Check sheet for the modelled part. Datum: model origin and axes. Units: mm. Face numbers are marked on the shaded views. A direction names the side the tool comes from. Coordinates: 2 decimals unless noted, no trailing zeros. Loops run counter-clockwise (first coordinate to the right, second up) from the corner with the lowest first, then second, coordinate; pieces in that order, holes last. Notation, with made-up numbers: (75.5, -1) - (91.5, -1) arc R18 cw to (91.5, 27) - close; hole circle Ø10 at (2, 0.5). An arc over 180 degrees is marked (long way). Use a Markdown table: item, result. Add a question column.
1) Sectioned sample at D-D, the plane x = 5.5. Enter the section's corners in (y, z).
2) Thickness scan on line 1 (X direction, y = -10.5, z = -4); line 2 (Y direction, x = 29, z = -2); line 3 (X direction, y = -14, z = -20). Record the ranges inside material, lowest first.
3) Sectioned sample at B-B, the plane z = -7. Enter the section's corners in (x, y), then the cut area to 3 significant figures.
4) Draft check along Z on the marked faces 1, 2 and 3. Enter one of: pulls with the +Z half, pulls with the -Z half, needs draft (parallel to the pull), parting line crosses it, or undercut.
5) Sectioned sample at C-C, the plane y = -8. State how many separate pieces and enclosed holes the cut face has, then the cut area to 3 significant figures.
6) Sectioned sample at A-A, the plane y = -16.5. Enter the section's corners in (x, z), then the cut area to 3 significant figures.
7) Tool access check on the marked faces 4, 5, 6 and 7. Record the directions out of +Z, -Z, +X, -X, +Y, -Y that give a thin tool (end or side, any length) a straight path to the whole face; none if there is none.
8) Go/stop test with flat-tipped pins: P1, Ø1.5, axis at x = -23, y = -9.5, coming from the +Z side; P2, Ø9.5, axis at x = 16, z = 0.5, coming from the -Y side; P3, Ø16.5, axis at x = 7.5, y = -5.5, coming from the -Z side. Record where each tip stops, or that it passes through.
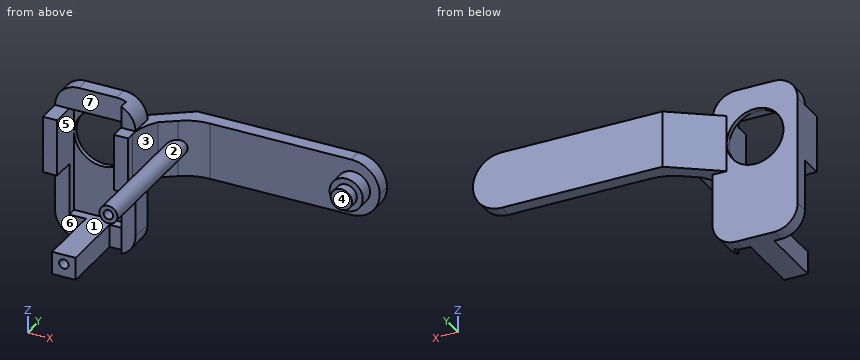
from build123d import *

# Parameters (mm, degrees)
SKETCH1_W            = 40
SKETCH1_H            = 12
BOSS_EXTRUDE1_DEPTH  = 3
SKETCH1_7_R          = 3.5
BOSS_EXTRUDE2_DEPTH  = 3
BOSS_EXTRUDE4_DEPTH  = 12
SKETCH4_W            = 3
SKETCH4_H            = 12
BOSS_EXTRUDE5_DEPTH  = 5
FILLET3_R            = 10
BOSS_EXTRUDE11_START = -27.8
BOSS_EXTRUDE11_DEPTH = 32.8
CUT_EXTRUDE2_DEPTH   = 47.899705007
FILLET7_R            = 6
BOSS_EXTRUDE12_DEPTH = 5
CUT_EXTRUDE3_START   = -2
CUT_EXTRUDE3_DEPTH   = 2
SKETCH13_W           = 3
SKETCH13_H           = 12
BOSS_EXTRUDE13_DEPTH = 5
SKETCH13_3_W         = 5
SKETCH13_3_H         = 4.8
BOSS_EXTRUDE14_DEPTH = 14
SKETCH14_R           = 1
CUT_EXTRUDE4_DEPTH   = 10
FILLET8_R            = 10
FILLET9_R            = 5
SKETCH15_R           = 1.9
SKETCH15_R_2         = 1
BOSS_EXTRUDE15_DEPTH = 30
SKETCH15_2_R         = 1
BOSS_EXTRUDE16_DEPTH = 20


# Read off the part's stored shape, not the designer's step: Boss-Extrude11, Cut-Extrude3
# Some blends are built 0.0001 mm under size
with BuildPart() as part:
    # Sketch1 → Boss-Extrude1 (new body)
    with BuildSketch(Plane(origin=(0, 0, 0), x_dir=(1, 0, 0), z_dir=(0, 1, 0))):
        with Locations((20.375241408, -0.133846421)):
            Rectangle(SKETCH1_W, SKETCH1_H)
    extrude(amount=BOSS_EXTRUDE1_DEPTH)

    # Sketch1<7> → Boss-Extrude2 (add)
    with BuildSketch(Plane(origin=(0, 0, 0), x_dir=(1, 0, 0), z_dir=(0, 1, 0))):
        with Locations(Location((34.817424324, -0.133846421, 0), (0, 0, 270))):
            Circle(SKETCH1_7_R)
    extrude(amount=-BOSS_EXTRUDE2_DEPTH)

    # Sketch3 → Boss-Extrude4 (add)
    with BuildSketch(Plane.XY.offset(6.133846421)):
        Polygon((0.375241408, 3), (-9.624758592, -4), (-4.393377613, -4), (5.606622387, 3), align=None)
    extrude(amount=-BOSS_EXTRUDE4_DEPTH)

    # Sketch4 → Boss-Extrude5 (add)
    with BuildSketch(Plane(origin=(0, -4, 0), x_dir=(-1, 0, 0), z_dir=(0, -1, 0))):
        with Locations((8.124758592, -0.133846421)):
            Rectangle(SKETCH4_W, SKETCH4_H)
    extrude(amount=BOSS_EXTRUDE5_DEPTH)

    # Fillet3
    fillet3_edges = [part.edges().sort_by_distance(p)[0] for p in [
        (1.320908101, 0, 0.133846421),
    ]]
    fillet(fillet3_edges, radius=FILLET3_R)

    # Boss-Extrude11 outline → Boss-Extrude11 (add)
    with BuildSketch(Plane.XY.offset(6.133846421).offset(BOSS_EXTRUDE11_START)):
        Polygon((-9.624758592, -7), (-9.624758592, -9), (-6.624758592, -9), (-6.624758592, -4), (-24.624758592, -4), (-24.624758592, -7), align=None)
    extrude(amount=BOSS_EXTRUDE11_DEPTH)

    # Sketch12 → Cut-Extrude2 (cut, through all)
    with BuildSketch(Plane(origin=(0, -7, 0), x_dir=(-1, 0, 0), z_dir=(0, -1, 0))):
        with BuildLine():
            ThreePointArc((9.624758592, -0.133846421), (11.382117904, -4.376487108), (15.624758592, -6.133846421))
            Line((15.624758592, -6.133846421), (15.624758592, 5.866153579))
            ThreePointArc((15.624758592, 5.866153579), (11.382117904, 4.108794266), (9.624758592, -0.133846421))
        make_face()
        with BuildLine():
            Line((15.624758592, 5.866153579), (15.624758592, -6.133846421))
            ThreePointArc((15.624758592, -6.133846421), (19.867399279, -4.376487108), (21.624758592, -0.133846421))
            ThreePointArc((21.624758592, -0.133846421), (19.867399279, 4.108794266), (15.624758592, 5.866153579))
        make_face()
    extrude(amount=-CUT_EXTRUDE2_DEPTH, mode=Mode.SUBTRACT)

    # Fillet7
    fillet7_edges = [part.edges().sort_by_distance(p)[0] for p in [
        (40.375241408, 1.5, -5.866153579),
        (40.375241408, 1.5, 6.133846421),
    ]]
    fillet(fillet7_edges, radius=FILLET7_R - 0.0001)  # a hair under: the kernel refuses the full size

    # Sketch1<9> → Boss-Extrude12 (add)
    with BuildSketch(Plane(origin=(0, 0, 0), x_dir=(1, 0, 0), z_dir=(0, 1, 0))):
        with BuildLine():
            ThreePointArc((32.567424324, -0.133846421), (34.817424324, -2.383846421), (37.067424324, -0.133846421))
            Line((37.067424324, -0.133846421), (32.567424324, -0.133846421))
        make_face()
        with BuildLine():
            Line((32.567424324, -0.133846421), (37.067424324, -0.133846421))
            ThreePointArc((37.067424324, -0.133846421), (34.817424324, 2.116153579), (32.567424324, -0.133846421))
        make_face()
    extrude(amount=-BOSS_EXTRUDE12_DEPTH)

    # Cut-Extrude3 outline → Cut-Extrude3 (cut)
    with BuildSketch(Plane(origin=(0, -7, 0), x_dir=(-1, 0, 0), z_dir=(0, -1, 0)).offset(CUT_EXTRUDE3_START)):
        with BuildLine():
            Line((21.624758592, 16.866153579), (9.624758592, 16.866153579))
            Line((9.624758592, 16.866153579), (9.624758592, -0.133846426))
            ThreePointArc((9.624758592, -0.133846426), (15.624758589, 5.866153579), (21.624758592, -0.133846421))
            Line((21.624758592, -0.133846421), (21.624758592, 16.866153579))
        make_face()
        with BuildLine():
            ThreePointArc((15.624758592, -6.133846421), (11.382117907, -4.37648711), (9.624758592, -0.133846426))
            Line((9.624758592, -0.133846426), (9.624758592, -6.133846421))
            Line((9.624758592, -6.133846421), (15.624758592, -6.133846421))
        make_face()
        with BuildLine():
            Line((21.624758592, -6.133846421), (21.624758592, -0.133846421))
            ThreePointArc((21.624758592, -0.133846421), (19.867399279, -4.376487108), (15.624758592, -6.133846421))
            Line((15.624758592, -6.133846421), (21.624758592, -6.133846421))
        make_face()
    extrude(amount=CUT_EXTRUDE3_DEPTH, mode=Mode.SUBTRACT)

    # Sketch13 → Boss-Extrude13 (add)
    with BuildSketch(Plane(origin=(0, -7, 0), x_dir=(-1, 0, 0), z_dir=(0, -1, 0))):
        with Locations((8.124758592, -0.133846421)):
            Rectangle(SKETCH13_W, SKETCH13_H)
        with Locations((23.124758592, -0.133846421)):
            Rectangle(SKETCH13_W, SKETCH13_H)
    extrude(amount=BOSS_EXTRUDE13_DEPTH)

    # Sketch13<3> → Boss-Extrude14 (add)
    with BuildSketch(Plane(origin=(0, -7, 0), x_dir=(-1, 0, 0), z_dir=(0, -1, 0))):
        with Locations((15.624758592, 19.266153579)):
            Rectangle(SKETCH13_3_W, SKETCH13_3_H)
    extrude(amount=BOSS_EXTRUDE14_DEPTH)

    # Sketch14 → Cut-Extrude4 (cut)
    with BuildSketch(Plane.XZ.offset(21)):
        with Locations((-15.624758592, -18.866153579)):
            Circle(SKETCH14_R)
        with Locations((-15.624758592, 8.133846421)):
            Circle(SKETCH14_R)
    extrude(amount=-CUT_EXTRUDE4_DEPTH, mode=Mode.SUBTRACT)

    # Fillet8
    # the kernel refuses this fillet: 10 mm, written as the material it adds along each edge
    with BuildSketch(Plane(origin=(-6.624758592, -4, -5.866153579), x_dir=(1, 0, 0), z_dir=(0, 0, 1))) as fillet8_piece_1:
        with BuildLine():
            CenterArc((10, -6.296710133), FILLET8_R, 140.974145336, 39.025854664)
            Line((0, -6.296710133), (0, 0))
            Line((0, 0), (2.231380978, 0))
        make_face()
    extrude(amount=12)

    # Fillet9
    fillet9_edges = [part.edges().sort_by_distance(p)[0] for p in [
        (-24.624758592, -5.5, -21.666153579),
        (-6.624758592, -6.5, -21.666153579),
        (-6.624758592, -6.5, 11.133846421),
        (-24.624758592, -5.5, 11.133846421),
    ]]
    fillet(fillet9_edges, radius=FILLET9_R - 0.0001)  # a hair under: the kernel refuses the full size

    # Sketch15 → Boss-Extrude15 (add)
    with BuildSketch(Plane(origin=(0, 0, 0), x_dir=(-1, 0, 0), z_dir=(0, -1, 0))):
        with Locations(Location((1.624758592, -0.133846421, 0), (0, 0, 258.977606014))):
            Circle(SKETCH15_R)
        with Locations(Location((1.624758592, -0.133846421, 0), (0, 0, 248.699103744))):
            Circle(SKETCH15_R_2, mode=Mode.SUBTRACT)
    extrude(amount=BOSS_EXTRUDE15_DEPTH)

    # Sketch15<2> → Boss-Extrude16 (add)
    with BuildSketch(Plane(origin=(0, 0, 0), x_dir=(-1, 0, 0), z_dir=(0, -1, 0))):
        with Locations(Location((1.624758592, -0.133846421, 0), (0, 0, 90))):
            Circle(SKETCH15_2_R)
    extrude(amount=BOSS_EXTRUDE16_DEPTH)


solid = part.part
Solved:
| question | item | result |
|---|---|---|
| 1 | outline | (0, -5.87) - (3, -5.87) - (3, 6.13) - (0, 6.13) - close |
| 2 | line 1 | x = -24.62 to -21.62, -9.62 to -6.62 |
| 2 | line 2 | y = 0 to 3 |
| 2 | line 3 | x = -18.12 to -13.12 |
| 3 | outline | (-24.62, -7) - (-21.62, -7) - (-21.62, -5) - (-9.62, -5) - (-9.62, -9) - (-6.62, -9) - (-6.62, -4) - (-24.62, -4) - close |
| 3 | area | 36.0 mm2 |
| 4 | face 1 | undercut |
| 4 | face 2 | parting line crosses it |
| 4 | face 3 | needs draft |
| 5 | separate pieces | 4 |
| 5 | enclosed holes | 0 |
| 5 | area | 163 mm2 |
| 6 | outline | (-18.12, -21.67) - (-13.12, -21.67) - (-13.12, -16.87) - (-18.12, -16.87) - close; circle Ø3.8 at (-1.62, 0.13); hole circle Ø2 at (-15.62, -18.87) |
| 6 | area | 32.2 mm2 |
| 7 | face 4 | +Z, -Z, +X, -Y |
| 7 | face 5 | -Y |
| 7 | face 6 | -Z, -X, -Y |
| 7 | face 7 | +Z, -X, -Y |
| 8 | P1 | stops at z = 6.13 |
| 8 | P2 | stops at y = 0 |
| 8 | P3 | stops at z = -5.87 |
